Verification items for the finished model (mm, model axes). Coordinates: 2 decimals unless noted, no trailing zeros. Order: outer loops, then holes, each group sorted by start corner. A loop starts at its lowest first (then second) coordinate and runs counter-clockwise, first axis right, second up. Notation, with made-up numbers: (-33.5, 21.25) -> (-0.5, 21.25) arc R19 cw to (-0.5, 35.25) -> close; hole circle Ø7 at (51, -13). An arc over 180 degrees is marked (long way). Write item = value, one per line. Start each with the question number.
from build123d import *

# Parameters (mm, degrees)
SKETCH3_R               = 5
CUT_EXTRUDE1_DEPTH      = 13.5000001
CUT_EXTRUDE1_DEPTH_BACK = 433.5000001


with BuildPart() as part:
    # Sweep-Thin1: sweep along a path in Sketch1
    with BuildLine(Plane(origin=(0, 0, 0), x_dir=(1, 0, 0), z_dir=(0, 1, 0))) as sweep_thin1_path:
        Line((0, 0), (-610, 0))
        ThreePointArc((-610, 0), (-638.284271247, 11.715728753), (-650, 40))
        Line((-650, 40), (-650, 380))
        ThreePointArc((-650, 380), (-638.284271247, 408.284271247), (-610, 420))
        Line((-610, 420), (0, 420))
    # Sketch2 → Sweep-Thin1 (sweep)
    with BuildSketch(Plane(origin=(0, 0, 0), x_dir=(0, 0, -1), z_dir=(1, 0, 0))):
        with BuildLine():
            Line((4.5, 12.5), (-4.5, 12.5))
            ThreePointArc((-4.5, 12.5), (-10.156854249, 10.156854249), (-12.5, 4.5))
            Line((-12.5, 4.5), (-12.5, -4.5))
            ThreePointArc((-12.5, -4.5), (-10.156854249, -10.156854249), (-4.5, -12.5))
            Line((-4.5, -12.5), (4.5, -12.5))
            ThreePointArc((4.5, -12.5), (10.156854249, -10.156854249), (12.5, -4.5))
            Line((12.5, -4.5), (12.5, 4.5))
            ThreePointArc((12.5, 4.5), (10.156854249, 10.156854249), (4.5, 12.5))
        make_face()
        with BuildLine():
            Line((4.5, 9.5), (-4.5, 9.5))
            ThreePointArc((-4.5, 9.5), (-8.035533906, 8.035533906), (-9.5, 4.5))
            Line((-9.5, 4.5), (-9.5, -4.5))
            ThreePointArc((-9.5, -4.5), (-8.035533906, -8.035533906), (-4.5, -9.5))
            Line((-4.5, -9.5), (4.5, -9.5))
            ThreePointArc((4.5, -9.5), (8.035533906, -8.035533906), (9.5, -4.5))
            Line((9.5, -4.5), (9.5, 4.5))
            ThreePointArc((9.5, 4.5), (8.035533906, 8.035533906), (4.5, 9.5))
        make_face(mode=Mode.SUBTRACT)
    sweep(path=sweep_thin1_path.line)

    # Sketch3 → Cut-Extrude1 (cut, two sides)
    with BuildSketch(Plane.XY) as cut_extrude1_sk:
        with Locations((-50, 0)):
            Circle(SKETCH3_R)
    extrude(amount=CUT_EXTRUDE1_DEPTH, mode=Mode.SUBTRACT)
    extrude(cut_extrude1_sk.sketch, amount=-CUT_EXTRUDE1_DEPTH_BACK, mode=Mode.SUBTRACT)


solid = part.part
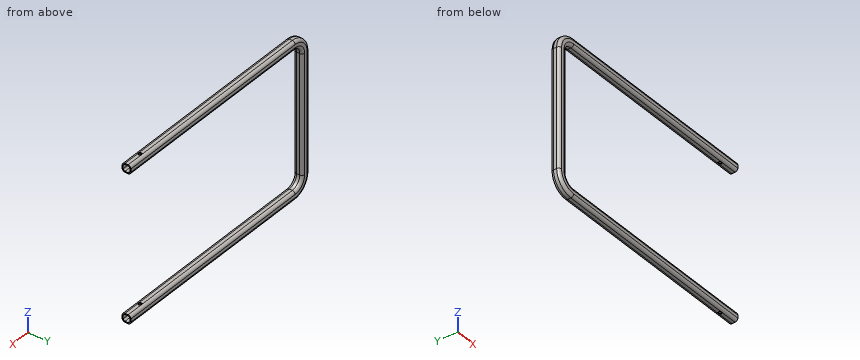
Item 1: Section check A-A (x = -402). State how many separate pieces and enclosed holes the cut face has, then the cut area to 3 significant figures.
Item 2: Section check B-B (z = -178.5). Record the boundary of the cut face in (x, y).
Item 3: Gauge pin test, flat ends, axial feed: P1, Ø11.5, axis at x = -50, y = 0, coming from the +Z side; P2, Ø6, axis at y = 4, z = -366, coming from the +X side. Record the tip position at first contact, or that the pin passes through.
Item 4: Thickness scan on line 1 (Z direction, x = -75.5, y = 4); line 2 (X direction, y = 4.5, z = -362); line 3 (Z direction, x = -509.5, y = 6). Record the ranges inside material, lowest first.
Filled sheet:
q1.separate_pieces = 2
q1.enclosed_holes = 2
q1.area = 461 mm^2
q2.outline = (-662.5, -4.5) arc R8 ccw to (-654.5, -12.5) -> (-645.5, -12.5) arc R8 ccw to (-637.5, -4.5) -> (-637.5, 4.5) arc R8 ccw to (-645.5, 12.5) -> (-654.5, 12.5) arc R8 ccw to (-662.5, 4.5) -> close; hole (-659.5, -4.5) arc R5 ccw to (-654.5, -9.5) -> (-645.5, -9.5) arc R5 ccw to (-640.5, -4.5) -> (-640.5, 4.5) arc R5 ccw to (-645.5, 9.5) -> (-654.5, 9.5) arc R5 ccw to (-659.5, 4.5) -> close
q3.P1 = 12.5
q3.P2 = -637.5
q4.line_1 = -432.5 to -429.5, -410.5 to -407.5, -12.5 to -9.5, 9.5 to 12.5
q4.line_2 = -662.5 to -659.5, -640.5 to -637.5
q4.line_3 = -432.36 to -429.27, -410.73 to -407.64, -12.36 to -9.27, 9.27 to 12.36
